Check sheet for the modelled part. Datum: model origin and axes. Units: mm. A direction names the side the tool comes from. Give positions to 0.01 mm unless a question says otherwise; leave off trailing zeros. Write each loop counter-clockwise with the first axis right and the second up, starting at its lowest first coordinate (ties: lowest second). Pieces come first, ordered by that corner, then holes. Notation, with made-up numbers: (12.5, 35) - (27.5, 35) arc R21 cw to (27.5, 47) - close; hole circle Ø3 at (-26.5, -17). An arc over 180 degrees is marked (long way). Return JSON: item names as keys, results as strings. Group by question number.
```python
from build123d import *

# Parameters (mm, degrees)
EXTRUDE_1_DEPTH     = 26
SKETCH_2_W          = 95
SKETCH_2_H          = 85
CUT_EXTRUDE_1_DEPTH = 23
SKETCH_3_W          = 96
SKETCH_3_H          = 86
CUT_EXTRUDE_2_DEPTH = 23
FILLET_1_R          = 1
FILLET_2_R          = 0.5


with BuildPart() as part:
    # Эскиз1 → Бобышка-Вытянуть1 (new body)
    with BuildSketch(Plane.XY):
        with BuildLine():
            Line((-48, -45), (48, -45))
            ThreePointArc((48, -45), (49.414213562, -44.414213562), (50, -43))
            Line((50, -43), (50, 43))
            ThreePointArc((50, 43), (49.414213562, 44.414213562), (48, 45))
            Line((48, 45), (-48, 45))
            ThreePointArc((-48, 45), (-49.414213562, 44.414213562), (-50, 43))
            Line((-50, 43), (-50, -43))
            ThreePointArc((-50, -43), (-49.414213562, -44.414213562), (-48, -45))
        make_face()
    extrude(amount=EXTRUDE_1_DEPTH)

    # Эскиз2 → Вырез-Вытянуть1 (cut)
    with BuildSketch(Plane(origin=(0, 0, 0), x_dir=(-1, 0, 0), z_dir=(0, 0, -1))):
        Rectangle(SKETCH_2_W, SKETCH_2_H)
    extrude(amount=-CUT_EXTRUDE_1_DEPTH, mode=Mode.SUBTRACT)

    # Эскиз3 → Вырез-Вытянуть2 (cut)
    with BuildSketch(Plane(origin=(0, 0, 0), x_dir=(-1, 0, 0), z_dir=(0, 0, -1))):
        Rectangle(SKETCH_3_W, SKETCH_3_H)
    extrude(amount=-CUT_EXTRUDE_2_DEPTH, mode=Mode.SUBTRACT)

    # Скругление1
    fillet_1_edges = [part.edges().sort_by_distance(p)[0] for p in [
        (48, 0, 23),
        (0, 43, 23),
        (-48, 0, 23),
        (0, -43, 23),
    ]]
    fillet(fillet_1_edges, radius=FILLET_1_R)

    # Скругление2
    fillet_2_edges = [part.edges().sort_by_distance(p)[0] for p in [
        (48, 0, 0),
        (0, -43, 0),
        (-48, 0, 0),
        (0, 43, 0),
    ]]
    fillet(fillet_2_edges, radius=FILLET_2_R)


solid = part.part
```
Item 1: Section check A-A on z = 4.75. Record the cut outline in (x, y).
Item 2: Section check C-C on y = -26.5. Record the cut outline in (x, z).
Item 3: Material ranges on line 1 along Y through (x, z) = (4, 4.5); line 2 along X through (y, z) = (15, 5.5); line 3 along Z through (x, y) = (44, -26), recorded low to high. Write a range as from..to.
Item 4: Mould release check, pull along X, two halves, no side actions. Record for faces 1 (the face through (1, 1, 23)), 2 (the face through (-50, 1, 13)), 3 (the face through (-1, 1, 26)): +X half, -X half, draft (parallel to the pull), parting line (faces both ways), or undercut.
Item 5: Section check B-B on x = 39. Record the cut outline in (y, z).
Item 6: Access from +Z, -Z, +X, -X, +Y, -Y to the whole of each face (thin tool, end or side, straight path). Record for faces 4 (the face through (1, -43, 11)), 5 (the face through (1, 45, 13)).
Item 7: Depth check by flat-ended pin: pin 1 (10 mm diameter, centred on x = -2, y = -12, fed in from -Z). Enter the tip coordinate at first touch or a pass-through.
Reply:
{
 "1": {"outline": "(-50, -43) arc R2 ccw to (-48, -45) - (48, -45) arc R2 ccw to (50, -43) - (50, 43) arc R2 ccw to (48, 45) - (-48, 45) arc R2 ccw to (-50, 43) - close; hole (-48, -43) - (48, -43) - (48, 43) - (-48, 43) - close"},
 "2": {"outline": "(-50, 0) - (-48.5, 0) arc R0.5 ccw to (-48, 0.5) - (-48, 22) arc R1 cw to (-47, 23) - (47, 23) arc R1 cw to (48, 22) - (48, 0.5) arc R0.5 ccw to (48.5, 0) - (50, 0) - (50, 26) - (-50, 26) - close"},
 "3": {"line 1": "-45..-43, 43..45", "line 2": "-50..-48, 48..50", "line 3": "23..26"},
 "4": {"face 1": "undercut", "face 2": "-X half", "face 3": "draft"},
 "5": {"outline": "(-45, 0) - (-43.5, 0) arc R0.5 ccw to (-43, 0.5) - (-43, 22) arc R1 cw to (-42, 23) - (42, 23) arc R1 cw to (43, 22) - (43, 0.5) arc R0.5 ccw to (43.5, 0) - (45, 0) - (45, 26) - (-45, 26) - close"},
 "6": {"face 4": "-Z", "face 5": "+Z, -Z, +X, -X, +Y"},
 "7": {"pin 1": "z = 23"}
}
